```python
from build123d import *

# Parameters (mm, degrees)
F1_DEPTH = 7.75
F2_R     = 1.25
F3_DEPTH = 10


with BuildPart() as f1:
    # F0 (on Front) → F1 (new body, symmetric)
    with BuildSketch(Plane.XZ):
        with BuildLine():
            Line((-1.25, 1.224745), (-1.25, -1.224745))
            ThreePointArc((-1.25, -1.224745), (0, -1.75), (1.25, -1.224745))
            Line((1.25, -1.224745), (1.25, 1.224745))
            ThreePointArc((1.25, 1.224745), (0, 1.75), (-1.25, 1.224745))
        make_face()
    extrude(amount=F1_DEPTH, both=True)

    # F2 (on Front) → F3 (join, symmetric)
    with BuildSketch(Plane.XZ):
        Circle(F2_R)
    extrude(amount=F3_DEPTH, both=True)


solid = f1.part
```
The model under review builds one solid part; all positions refer to its coordinate system, in mm. A direction names the side the tool comes from. Round coordinates to 2 decimals unless told otherwise and drop trailing zeros. Order: outer loops, then holes, each group sorted by start corner. A loop starts at its lowest first (then second) coordinate and runs counter-clockwise, first axis right, second up. Notation, with made-up numbers: M 33,87.25 L 87,87.25 A19 cw 87,92.25 Z; hole C 16,16.5 d2. An arc over 180 degrees is marked long. Use a Markdown table: item, result.
1) Insertion check: pin 1 (0.5 mm diameter, centred on x = 0.5, z = -1.5, fed in from +Y). The pin has a flat end and moves straight along its axis. Give the tip position at first contact, or say it passes through.
Report:
| item | result |
|---|---|
| pin 1 | y = 7.75 |
2) Consider section A-A (x = 0). Write out the cut boundary in (y, z), then the cut area to 3 significant figures.
Report:
| item | result |
|---|---|
| outline | M -10,-1.25 L -7.75,-1.25 L -7.75,-1.75 L 7.75,-1.75 L 7.75,-1.25 L 10,-1.25 L 10,1.25 L 7.75,1.25 L 7.75,1.75 L -7.75,1.75 L -7.75,1.25 L -10,1.25 Z |
| area | 65.5 mm^2 |
3) Tool access review of faces 1 (the face through (-0.01, 7.75, 1.4)), 2 (the face through (-0.01, -7.75, 1.4)), 3 (the face through (-0.1, -7.75, -1.4)), 4 (the face through (-0.27, -8.89, -1.22)): name each direction out of +Z, -Z, +X, -X, +Y, -Y from which nothing blocks a thin tool from reaching the whole face with its end or side.
Report:
| item | result |
|---|---|
| face 1 | +Z, +Y |
| face 2 | +Z, -Y |
| face 3 | -Z, -Y |
| face 4 | -Y |
4) Wall thickness on line 1 along Y through (x, z) = (-0.3, 1.5); line 2 along X through (y, z) = (-3, 1.25); line 3 along Z through (x, y) = (-0.1, 5.25): over which ranges is each line inside the solid? List them lowest first. Write a range as [from, to].
Report:
| item | result |
|---|---|
| line 1 | [-7.75, 7.75] |
| line 2 | [-1.22, 1.22] |
| line 3 | [-1.75, 1.75] |
5) Consider section C-C (z = -0.6). Write out the cut boundary in (x, y).
Report:
| item | result |
|---|---|
| outline | M -1.25,-7.75 L -1.1,-7.75 L -1.1,-10 L 1.1,-10 L 1.1,-7.75 L 1.25,-7.75 L 1.25,7.75 L 1.1,7.75 L 1.1,10 L -1.1,10 L -1.1,7.75 L -1.25,7.75 Z |
6) Consider section B-B (y = -8.25). Write out the cut boundary in (x, z).
Report:
| item | result |
|---|---|
| outline | C 0,0 d2.5 |
